```python
from build123d import *

# Parameters (mm, degrees)
CROQUIS1_R              = 4
CROQUIS1_R_2            = 5.75
CROQUIS1_R_3            = 4.05
SALIENTE_EXTRUIR1_DEPTH = 5
CROQUIS3_W              = 93.333333333
CROQUIS3_H              = 5
CORTAR_EXTRUIR1_DEPTH   = 10
CROQUIS6_R              = 2.5
CORTAR_EXTRUIR2_DEPTH   = 10


with BuildPart() as part:
    # Croquis1 → Saliente-Extruir1 (new body)
    with BuildSketch(Plane.XY):
        with BuildLine():
            Line((-125.472429705, -88.332065653), (154.527570295, -88.332065653))
            ThreePointArc((154.527570295, -88.332065653), (175.740773731, -79.545269088), (184.527570295, -58.332065653))
            Line((184.527570295, -58.332065653), (184.527570295, 81.667934347))
            ThreePointArc((184.527570295, 81.667934347), (175.740773731, 102.881137783), (154.527570295, 111.667934347))
            Line((154.527570295, 111.667934347), (-125.472429705, 111.667934347))
            ThreePointArc((-125.472429705, 111.667934347), (-146.68563314, 102.881137783), (-155.472429705, 81.667934347))
            Line((-155.472429705, 81.667934347), (-155.472429705, -58.332065653))
            ThreePointArc((-155.472429705, -58.332065653), (-146.68563314, -79.545269088), (-125.472429705, -88.332065653))
        make_face()
        with Locations((-105.472429705, 61.667934347)):
            Circle(CROQUIS1_R, mode=Mode.SUBTRACT)
        with Locations((-55.472429705, 71.667934347)):
            Circle(CROQUIS1_R, mode=Mode.SUBTRACT)
        with Locations((-55.472429705, 51.167934347)):
            Circle(CROQUIS1_R, mode=Mode.SUBTRACT)
        with Locations((144.027570295, -13.332065653)):
            Circle(CROQUIS1_R, mode=Mode.SUBTRACT)
        with Locations((164.527570295, -13.332065653)):
            Circle(CROQUIS1_R, mode=Mode.SUBTRACT)
        with Locations((144.027570295, 71.667934347)):
            Circle(CROQUIS1_R, mode=Mode.SUBTRACT)
        with Locations((164.527570295, 71.667934347)):
            Circle(CROQUIS1_R, mode=Mode.SUBTRACT)
        with Locations((-99.972429705, 91.667934347)):
            Circle(CROQUIS1_R, mode=Mode.SUBTRACT)
        with Locations((-120.472429705, 91.667934347)):
            Circle(CROQUIS1_R, mode=Mode.SUBTRACT)
        with Locations((-5.472429705, 50.667934347)):
            Circle(CROQUIS1_R_2, mode=Mode.SUBTRACT)
        with Locations((106.527570295, -45.332065653)):
            Circle(CROQUIS1_R_3, mode=Mode.SUBTRACT)
    extrude(amount=SALIENTE_EXTRUIR1_DEPTH)

    # Croquis3 → Cortar-Extruir1 (cut)
    with BuildSketch(Plane.XY.offset(5)):
        with Locations((14.527570296, -85.832065653)):
            Rectangle(CROQUIS3_W, CROQUIS3_H)
    extrude(amount=-CORTAR_EXTRUIR1_DEPTH, mode=Mode.SUBTRACT)

    # Croquis6 → Cortar-Extruir2 (cut)
    with BuildSketch(Plane.XY.offset(5)):
        with Locations((-78.805763038, -85.842065653)):
            Circle(CROQUIS6_R)
        with Locations((107.860903629, -85.842065653)):
            Circle(CROQUIS6_R)
    extrude(amount=-CORTAR_EXTRUIR2_DEPTH, mode=Mode.SUBTRACT)


solid = part.part
```
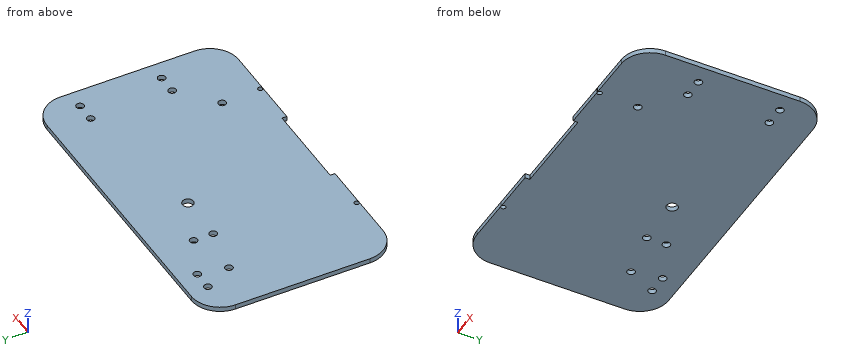
Model file for the job. Use its own axes, mm. Coordinates: 2 decimals unless noted, no trailing zeros. Order: outer loops, then holes, each group sorted by start corner. A loop starts at its lowest first (then second) coordinate and runs counter-clockwise, first axis right, second up. Notation, with made-up numbers: (49.5, -0.5) -> (83.5, -0.5) arc R21 cw to (83.5, 9.5) -> close; hole circle Ø4 at (15, -9). An arc over 180 degrees is marked (long way). Answer as a JSON object with one key per item and string values. Group by question number.
1) Cut at B-B, the plane x = -120.5. Write the cut outline in (y, z).
2) Cut at A-A, the plane z = 2.75. Count the separate pieces of the cut face and the enclosed holes in it, then the cut area to 3 significant figures.
3) Cut at C-C, the plane x = 26.5. Write the cut outline in (y, z).
4) Drill centre lines: L1, parallel to Y at x = 141.5, z = 1.75; L2, parallel to Y at x = -100, z = 1.6; L3, parallel to Y at x = -3, z = 3.3. Where is each one in solid material? Low to high.
5) Flat gauge pins, fed straight in: pin 1 (1.5 mm diameter, centred on y = -86, z = 3, fed in from +X); pin 2 (10.5 mm diameter, centred on x = -55.47, y = 51.17, fed in from +Z). Where does each tip first touch, or does it go through?
Check values:
{
 "1": {"outline": "(-88.33, 0) -> (87.67, 0) -> (87.67, 5) -> (-88.33, 5) -> close; (95.67, 0) -> (111.67, 0) -> (111.67, 5) -> (95.67, 5) -> close"},
 "2": {"separate pieces": "1", "enclosed holes": "11", "area": "66,100 mm²"},
 "3": {"outline": "(-83.33, 0) -> (111.67, 0) -> (111.67, 5) -> (-83.33, 5) -> close"},
 "4": {"L1": "y = -88.33 to -16.43, -10.23 to 68.57, 74.77 to 111.67", "L2": "y = -88.33 to 87.67, 95.67 to 111.67", "L3": "y = -83.33 to 45.48, 55.86 to 111.67"},
 "5": {"pin 1": "stops at x = 167.77", "pin 2": "stops at z = 5"}
}
